Answer from the drawing. Dimensions are ordinates in mm from the lowest x, y and z of the part. Round coordinates to 2 decimals unless told otherwise and drop trailing zeros. Write each loop counter-clockwise with the first axis right and the second up, starting at its lowest first coordinate (ties: lowest second). Pieces come first, ordered by that corner, then holes. Notation, with made-up numbers: (87, 66) - (146, 66) arc R34 cw to (146, 100) - close; hole circle Ø1 at (55.5, 23.25). An arc over 180 degrees is marked (long way). Answer in a Markdown table with one row per item.
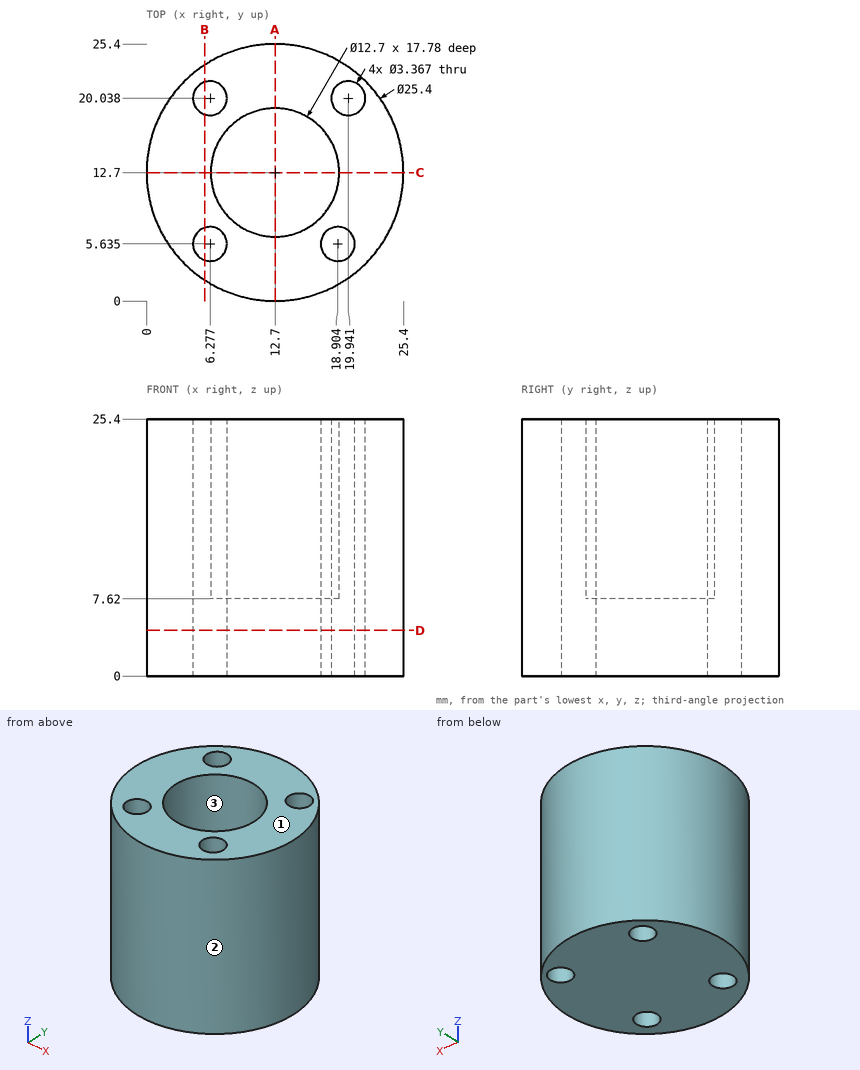
(1) For a pull along X with two mould halves and no side action, classify the marked faces 1, 2 and 3 as pulls with the +X half, pulls with the -X half, needs draft (parallel to the pull), parting line crosses it, or undercut.
Checked values:
| item | result |
|---|---|
| face 1 | needs draft |
| face 2 | parting line crosses it |
| face 3 | undercut |
(2) Section B-B (x = 5.75) is taken. Give the vertices of the cut face in (y, z) (1 decimal).
Checked values:
| item | result |
|---|---|
| outline | (2.1, 0) - (4, 0) - (4, 25.4) - (2.1, 25.4) - close; (7.2, 0) - (18.4, 0) - (18.4, 25.4) - (7.2, 25.4) - close; (21.6, 0) - (23.3, 0) - (23.3, 25.4) - (21.6, 25.4) - close |
(3) Section D-D (z = 4.5) is taken. Give the vertices of the cut face in (x, y) (1 decimal), and give its area (3 significant figures).
Checked values:
| item | result |
|---|---|
| outline | circle Ø25.4 at (12.7, 12.7); hole circle Ø3.4 at (6.3, 5.6); hole circle Ø3.4 at (6.3, 20); hole circle Ø3.4 at (18.9, 5.6); hole circle Ø3.4 at (19.9, 20) |
| area | 471 mm2 |
(4) Find the intervals of material crossed by line 1 (Y direction, x = 12.7, z = 14.25); line 2 (X direction, y = 5.25, z = 11) (1 decimal); line 3 (Y direction, x = 7.5, z = 16.5) (1 decimal), in increasing order.
Checked values:
| item | result |
|---|---|
| line 1 | y = 0 to 6.35, 19.05 to 25.4 |
| line 2 | x = 2.4 to 4.6, 7.9 to 17.3, 20.5 to 23 |
| line 3 | y = 1.1 to 4.5, 6.8 to 9.1, 16.3 to 18.9, 21.2 to 24.3 |
(5) Flat-ended cylindrical pins translate along their axes: pin 1 (4 mm diameter, centred on y = 6.5, z = 10.5, fed in from +X) (1 decimal); pin 2 (1 mm diameter, centred on y = 8, z = 4.5, fed in from -X) (1 decimal); pin 3 (6 mm diameter, centred on y = 19.5, z = 20.5, fed in from -X). Find the tip coordinate at first contact, or state that the pin passes through.
Checked values:
| item | result |
|---|---|
| pin 1 | stops at x = 24.7 |
| pin 2 | stops at x = 0.7 |
| pin 3 | stops at x = 0.58 |
(6) Section A-A (x = 12.7) is taken. Give the vertices of the cut face in (y, z), and give its area (3 significant figures).
Checked values:
| item | result |
|---|---|
| outline | (0, 0) - (25.4, 0) - (25.4, 25.4) - (19.05, 25.4) - (19.05, 7.62) - (6.35, 7.62) - (6.35, 25.4) - (0, 25.4) - close |
| area | 419 mm2 |
